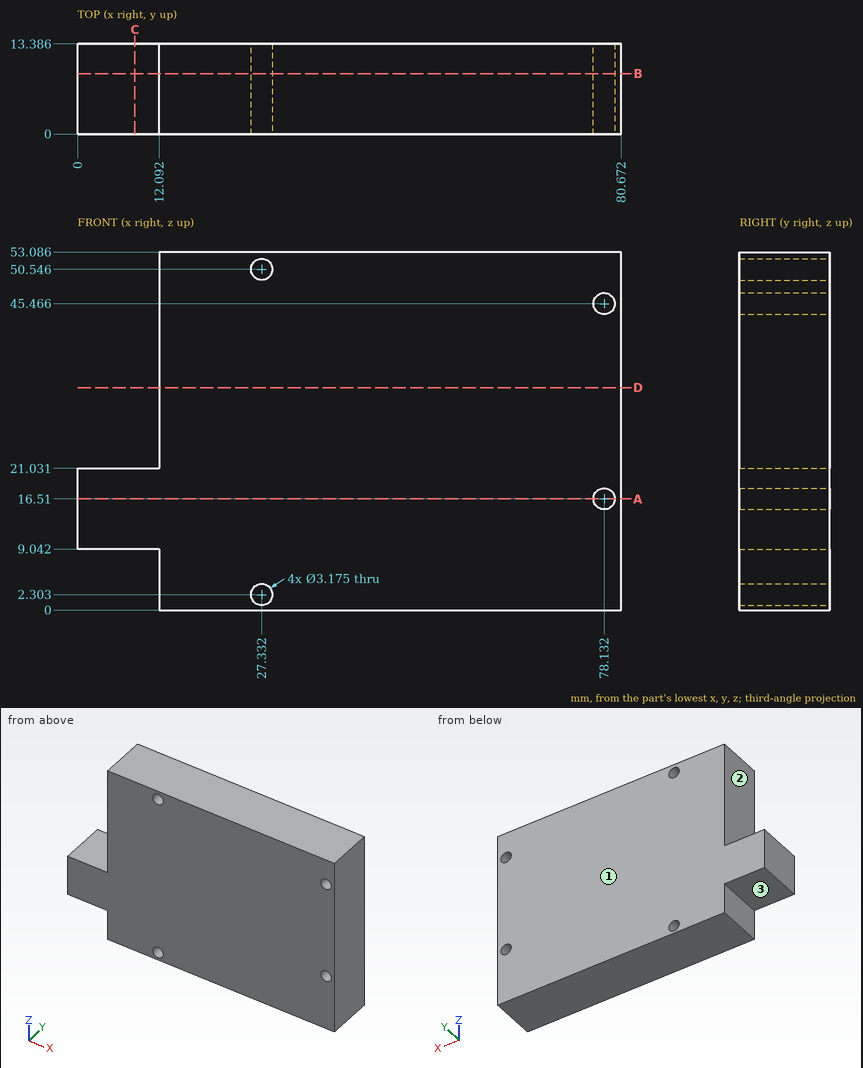
Check sheet for the drawn part. Datum: minimum x, y, z corner. Units: mm. A direction names the side the tool comes from. Round coordinates to 2 decimals unless told otherwise and drop trailing zeros. Order: outer loops, then holes, each group sorted by start corner. A loop starts at its lowest first (then second) coordinate and runs counter-clockwise, first axis right, second up. Notation, with made-up numbers: (74.25, 68.5) -> (130.25, 68.5) arc R27 ccw to (130.25, 106.5) -> close; hole circle Ø8 at (-33, 23). An arc over 180 degrees is marked (long way). Use CSV: the item, a comma, the result in double quotes.
(1) Tool access check on the marked faces 1, 2 and 3. Record the directions out of +Z, -Z, +X, -X, +Y, -Y that give a thin tool (end or side, any length) a straight path to the whole face; none if there is none.
Worked out:
face 1,"+Z, -Z, +X, -X, +Y"
face 2,"+Z, -X, +Y, -Y"
face 3,"-Z, -X, +Y, -Y"
(2) Depth check by flat-ended pin: pin 1 (3.5 mm diameter, centred on x = 6.5, y = 7, fed in from +Z); pin 2 (3 mm diameter, centred on y = 4.5, z = 29.5, fed in from -X). Enter the tip coordinate at first touch or a pass-through.
Worked out:
pin 1,"z = 21.03"
pin 2,"x = 12.09"
(3) Cross-section at A-A (z = 16.51). Record the boundary of the cut face in (x, y) (1 decimal).
Worked out:
outline,"(0, 0) -> (76.5, 0) -> (76.5, 13.4) -> (0, 13.4) -> close; (79.7, 0) -> (80.7, 0) -> (80.7, 13.4) -> (79.7, 13.4) -> close"
(4) Cross-section at D-D (z = 33). Record the boundary of the cut face in (x, y) (1 decimal).
Worked out:
outline,"(12.1, 0) -> (80.7, 0) -> (80.7, 13.4) -> (12.1, 13.4) -> close"
(5) Cross-section at B-B (y = 9). Record the boundary of the cut face in (x, z) (1 decimal).
Worked out:
outline,"(0, 9) -> (12.1, 9) -> (12.1, 0) -> (80.7, 0) -> (80.7, 53.1) -> (12.1, 53.1) -> (12.1, 21) -> (0, 21) -> close; hole circle Ø3.2 at (27.3, 2.3); hole circle Ø3.2 at (27.3, 50.5); hole circle Ø3.2 at (78.1, 16.5); hole circle Ø3.2 at (78.1, 45.5)"
(6) Material ranges on line 1 along X through (y, z) = (6.25, 16.51) (1 decimal); line 2 along X through (y, z) = (10.5, 34); line 3 along X through (y, z) = (10.75, 44.5), recorded low to high. Write a range as from..to.
Worked out:
line 1,"0..76.5, 79.7..80.7"
line 2,"12.09..80.67"
line 3,"12.09..76.87, 79.39..80.67"
(7) Cross-section at C-C (x = 8.5). Record the boundary of the cut face in (y, z) (1 decimal).
Worked out:
outline,"(0, 9) -> (13.4, 9) -> (13.4, 21) -> (0, 21) -> close"
